from build123d import *

# Parameters (mm, degrees)
F0_R      = 14
F0_R_2    = 3.25
F1_DEPTH  = 7
F2_R      = 13
F3_DEPTH  = 5
F5_DEPTH  = 7
F6_W      = 8.5
F6_H      = 2
F7_DEPTH  = 12.8
F8_W      = 6.5
F8_H      = 5
F9_DEPTH  = 17.5
F10_W     = 1
F10_H     = 5
F11_DEPTH = 0.5
F12_W     = 1
F12_H     = 5
F13_DEPTH = 0.5
F14_SIZE  = 0.49999
F15_SIZE  = 1


# Not quite as in the source:
# - a fillet or chamfer is up to 0.001 mm smaller than in the source, because OpenCascade refuses the exact size


with BuildPart() as f1:
    # F0 (on Top) → F1 (new body)
    with BuildSketch(Plane.XY):
        Circle(F0_R)
        Circle(F0_R_2, mode=Mode.SUBTRACT)
    extrude(amount=F1_DEPTH)

    # F2 (on face) → F3 (cut)
    with BuildSketch(Plane.XY.offset(7)):
        Circle(F2_R)
    extrude(amount=-F3_DEPTH, mode=Mode.SUBTRACT)

    # F4 (on face) → F5 (join)
    with BuildSketch(Plane.XY.offset(7)):
        with BuildLine():
            Line((-14, 17.5), (-14, 0))
            ThreePointArc((-14, 0), (-13.7477270849, 2.6457513111), (-13, 5.1961524227))
            Line((-13, 5.1961524227), (-13, 17.5))
            Line((-13, 17.5), (-14, 17.5))
        make_face()
        with BuildLine():
            ThreePointArc((-6.5, 12.3995967676), (-6.0046946559, 12.6468827024), (-5.5, 12.8743931896))
            Line((-5.5, 12.8743931896), (-5.5, 17.5))
            Line((-5.5, 17.5), (-6.5, 17.5))
            Line((-6.5, 17.5), (-6.5, 12.3995967676))
        make_face()
    extrude(amount=-F5_DEPTH)

    # F6 (on face) → F7 (join)
    with BuildSketch(Plane(origin=(0, 17.5, 0), x_dir=(-1, 0, 0), z_dir=(0, 1, 0))):
        with Locations((9.75, 1)):
            Rectangle(F6_W, F6_H)
    extrude(amount=-F7_DEPTH)

    # F8 (on face) → F9 (cut)
    with BuildSketch(Plane(origin=(0, 17.5, 0), x_dir=(-1, 0, 0), z_dir=(0, 1, 0))):
        with Locations((9.75, 4.5)):
            Rectangle(F8_W, F8_H)
    extrude(amount=-F9_DEPTH, mode=Mode.SUBTRACT)

    # F10 (on face) → F11 (join)
    with BuildSketch(Plane.YZ.offset(-13)):
        with Locations((0.5, 4.5)):
            Rectangle(F10_W, F10_H)
        with Locations((17, 4.5)):
            Rectangle(F10_W, F10_H)
    extrude(amount=F11_DEPTH)

    # F12 (on face) → F13 (join)
    with BuildSketch(Plane(origin=(-6.5, 0, 0), x_dir=(0, -1, 0), z_dir=(-1, 0, 0))):
        with Locations((-17, 4.5)):
            Rectangle(F12_W, F12_H)
    extrude(amount=F13_DEPTH)

    # F14 (size 0.5 in the source; OpenCascade refuses exactly that, so slightly less here)
    f14_edges = [f1.edges().sort_by_distance(p)[0] for p in [
        (-12.5, 0.5, 7),
        (-12.5, 17, 7),
        (-7, 17, 7),
    ]]
    chamfer(f14_edges, length=F14_SIZE)

    # F15
    f15_edges = [f1.edges().sort_by_distance(p)[0] for p in [
        (11.683321, -7.713624, 0),
        (-5.5, 15.187197, 0),
        (-14, 8.75, 0),
    ]]
    chamfer(f15_edges, length=F15_SIZE)


solid = f1.part
Can you work these out from the model? Positions are in its coordinate system, mm. A direction names the side the tool comes from. Round coordinates to 2 decimals unless told otherwise and drop trailing zeros. Loops run counter-clockwise (first coordinate to the right, second up) from the corner with the lowest first, then second, coordinate; pieces in that order, holes last. Notation, with made-up numbers: (82, -24.5) - (136, -24.5) arc R20 cw to (136, -18.5) - close; hole circle Ø11 at (18.5, 1). An arc over 180 degrees is marked (long way). Answer in a Markdown table with one row per item. Add a question column.
Q1. I want a section at B-B on z = 5.5. List the corners of the cut face in (x, y) for me, and give its area (3 significant figures).
Q2. Which directions (+Z, -Z, +X, -X, +Y, -Y) give clear straight access to the entire face, cutting with the end or side of a thin tool? Please do faces 4 (the cylindrical face through (11.01, -6.91, 4.54)), 5 (the flat face through (-6, 15, 0.5)), 6 (the flat face through (-5.5, 15, 4)), 7 (the conical face through (11.16, -7, 0.174)), 8 (the flat face through (-12.5, 17, 4)).
Q3. We'd pull the mould along X, two halves only. Please class faces 1 (the flat face through (-14, 9, 4)), 2 (the flat face through (-6.5, 14, 5)), 3 (the flat face through (-10, 17.5, 1)): pulls with the +X half, pulls with the -X half, needs draft (parallel to the pull), parting line crosses it, or undercut.
Q4. I need wall thicknesses on L1, parallel to Y at x = 0, z = 5.9; L2, parallel to Y at x = 0, z = 1.3; L3, parallel to Z at x = -6.75, y = -2. Which ranges of each line are inside material? Lowest first, please.
Q5. For pin 1 Ø5 at (x, y) = (2, -8) entering from +Z; pin 2 Ø1.5 at (x, z) = (8.5, 3) entering from +Y; pin 3 Ø4 at (x, z) = (5, 4.5) entering from -Y, each with a flat end and sliding along its axis, tell me the tip position at first contact or that it passes through.
Q6. I want a section at A-A on x = 0. List the corners of the cut face in (y, z) for me.
Q7. I want a section at C-C on z = 0.5. List the corners of the cut face in (x, y) for me.
A:
| question | item | result |
|---|---|---|
| 1 | outline | (-14, 0) arc R14 ccw (long way) to (-5.5, 12.87) - (-5.5, 17.5) - (-7, 17.5) - (-7, 16.5) - (-6.5, 16.5) - (-6.5, 11.26) arc R13 cw (long way) to (-13, 0) - (-12.5, 0) - (-12.5, 1) - (-13, 1) - (-13, 16.5) - (-12.5, 16.5) - (-12.5, 17.5) - (-14, 17.5) - close |
| 1 | area | 94.3 mm^2 |
| 2 | face 4 | +Z |
| 2 | face 5 | -Z, +Y |
| 2 | face 6 | +Z, -Z, +Y |
| 2 | face 7 | -Z |
| 2 | face 8 | +Z, +Y |
| 3 | face 1 | pulls with the -X half |
| 3 | face 2 | undercut |
| 3 | face 3 | needs draft |
| 4 | L1 | -14 to -13, 13 to 14 |
| 4 | L2 | -14 to -3.25, 3.25 to 14 |
| 4 | L3 | 0 to 2 |
| 5 | pin 1 | z = 2 |
| 5 | pin 2 | y = 11.66 |
| 5 | pin 3 | y = -13.67 |
| 6 | outline | (-14, 1) - (-13, 0) - (-3.25, 0) - (-3.25, 2) - (-13, 2) - (-13, 7) - (-14, 7) - close; (3.25, 0) - (13, 0) - (14, 1) - (14, 7) - (13, 7) - (13, 2) - (3.25, 2) - close |
| 7 | outline | (-13.5, 0) arc R13.5 ccw (long way) to (-6, 12.09) - (-6, 17.5) - (-13.5, 17.5) - close; hole circle Ø6.5 at (0, 0) |
